Verification items for the finished model (mm, model axes). A direction names the side the tool comes from. Give positions to 0.01 mm unless a question says otherwise; leave off trailing zeros. Write each loop counter-clockwise with the first axis right and the second up, starting at its lowest first coordinate (ties: lowest second). Pieces come first, ordered by that corner, then holes. Notation, with made-up numbers: M -27,-3.5 L 19,-3.5 A23 ccw 19,9.5 Z; hole C 37,10 d7. An arc over 180 degrees is marked long. Answer as a JSON object with one key per item and string values.
Autodesk Fusion 360 part; units mm, degrees
sketch "Sketch1" plane through (0, 0, 0) normal (0, 0, 1) x (1, 0, 0)
  line L0 (36, 27) -> (-36, 27)
  line L1 (-36, 27) -> (-36, -27)
  line L2 (-36, -27) -> (36, -27)
  line L3 (36, -27) -> (36, 27)
  line L4 (36, 30.6) -> (-36, 30.6)
  line L5 (-36, 35.6) -> (-36, -30.6)
  line L6 (-36, -30.6) -> (36, -30.6)
  line L7 (36, -30.6) -> (36, 30.6)
  line L8 (33, 35.6) -> (-36, 35.6)
  line L9 (41, -27.6) -> (41, 27.6)
  line L10 (33, -35.6) -> (-36, -35.6)
  line L11 (-36, -35.6) -> (-36, 30.6)
  arc A0 (41, 27.6) -> (33, 35.6) centre (33, 27.6) ccw
  arc A1 (33, -35.6) -> (41, -27.6) centre (33, -27.6) ccw
  circle A2 centre (-31, 0) radius 1.75
  line L12 (-31, 11) -> (-10, 11)
  arc A3 (-10, 11) -> (-10, 19) centre (-10, 15) ccw
  line L13 (-10, 19) -> (-31, 19)
  arc A4 (-31, 19) -> (-31, 11) centre (-31, 15) ccw
  line L14 (-31, 15) -> (-10, 15) construction
  line L15 (1.75, 0) -> (22.5, 0)
  line L16 (-31, -11) -> (-10, -11)
  line L17 (-10, -19) -> (-31, -19)
  arc A5 (-10, -19) -> (-10, -11) centre (-10, -15) ccw
  arc A6 (-31, -11) -> (-31, -19) centre (-31, -15) ccw
  circle A7 centre (-10, 0) radius 1.75
  dimension "d1" = 72
  dimension "d2" = 54
  dimension "d3" = 61.2
  dimension "d6" = 8
  dimension "d32" = 3.5
  dimension "d34" = 8
  dimension "d40" = 3.5
extrude "Extrude1" add sketch "Sketch1" along normal blind 6.1 contours L3 L4 L5 L6 L7 L8 L9 L10 L11 A0 A1 | L0 L4 L5 L7 L11 | L2 L5 L6 L7 L11
extrude "Extrude2" add sketch "Sketch1" along normal blind 24 contours L3 L4 L5 L6 L7 L8 L9 L10 L11 A0 A1
extrude "Extrude3" add sketch "Sketch1" along normal blind 27 and the other way blind -24
sketch "Sketch2" plane through (0, -35.6, 0) normal (0, -1, 0) x (1, 0, 0)
  line L0 (-36, 0) -> (33, 0)
  line L1 (33, 0) -> (33, 27)
  line L2 (-36, 27) -> (-36, 0)
  line L3 (-36, 0) -> (-49.5029, 27)
  line L4 (-36, 0) -> (-6, 0) construction
  line L5 (-36, 27) -> (-49.5029, 27)
  line L6 (33, 27) -> (-36, 27)
  line L7 (-36, 27) -> (-36, 24)
  line L8 (-36, 24) -> (-36.4845, 24)
  line L9 (-36.4845, 24) -> (-48.0026, 24)
  line L10 (-36, 0) -> (-36, 6.4)
  line L11 (-36, 6.4) -> (-36, 6)
  line L12 (-36, 6.4) -> (-39.2007, 6.4)
  line L13 (-36, 0) -> (-32.4, 0)
  line L14 (-49.5029, 27) -> (-47.5029, 27)
  line L15 (-36, 6.4) -> (-32.4, 6.4)
  line L16 (-32.4, 6.4) -> (-32.4, 0)
  dimension "d11" = 116.57
  dimension "d25" = 6.4
  dimension "d36" = 3.6
  dimension "d37" = 2
extrude "Extrude4" add sketch "Sketch2" against normal blind 5 contours L2 L3 L10 L11 L12 | L2 L3 L8 L9 L12
extrude "Extrude5" add sketch "Sketch2" along normal blind -71.2 and the other way blind 66.2 contours L2 L3 L10 L11 L12 | L2 L3 L8 L9 L12
extrude "Extrude6" add sketch "Sketch2" against normal blind 71.2 contours L2 L3 L5 L7 L8 L9 L14
extrude "Extrude7" cut sketch "Sketch2" along normal blind -8.6 and the other way blind 5 contours L0 L2 L10 L11 L13 L15 L16
extrude "Extrude8" cut sketch "Sketch2" along normal blind -66.2 and the other way blind 62.6 contours L0 L2 L10 L11 L13 L15 L16
chamfer "Chamfer2" distance 1 angle 45 2 edges at (-32.6316, 0.6328, 24) (-11.6316, 0.6328, 24)
sketch "Sketch3" plane through (0, 0, 27) normal (0, 0, 1) x (-1, 0, 0)
  arc A0 (10, 19) -> (10, 11) centre (10, 15) ccw
  line L0 (10, 19) -> (31, 19)
  arc A1 (31, 11) -> (31, 19) centre (31, 15) ccw
  line L1 (31, 11) -> (10, 11)
  circle A2 centre (31, 0) radius 1.75
  circle A3 centre (10, 0) radius 1.75
  arc A4 (31, -19) -> (31, -11) centre (31, -15) ccw
  line L2 (31, -19) -> (10, -19)
  arc A5 (10, -11) -> (10, -19) centre (10, -15) ccw
  line L3 (10, -11) -> (31, -11)
  line L4 (49.5029, 35.6) -> (-33, 35.6)
  arc A6 (-33, 35.6) -> (-41, 27.6) centre (-33, 27.6) ccw
  line L5 (-41, 27.6) -> (-41, -27.6)
  arc A7 (-41, -27.6) -> (-33, -35.6) centre (-33, -27.6) ccw
  line L6 (-33, -35.6) -> (49.5029, -35.6)
  line L7 (49.5029, -35.6) -> (49.5029, 35.6)
  line L8 (2.0837, -40) -> (-45, -40)
  line L9 (-45, -40) -> (-45, 40)
  line L10 (-45, 40) -> (2.0837, 40)
  line L11 (2.0837, 40) -> (2.0837, -40)
extrude "Extrude9" cut sketch "Sketch3" against normal blind 55 contours L4 A6 L5 A7 L6 L11 | L4 A6 L5 A7 L6 L8 L9 L10 L11
chamfer "Chamfer3" distance 1 angle 45 2 edges at (-32.4, -28.8, 6.1) (-32.4, 28.8, 6.1)
1) Thickness scan on L1, parallel to Y at x = -31, z = 26.15; L2, parallel to Y at x = -37.5, z = 16; L3, parallel to Y at x = -17, z = 3.5. Record the ranges inside material, lowest first.
Completed:
{"L1": "y = -35.6 to -19, -11 to -1.75, 1.75 to 11, 19 to 35.6", "L2": "y = -35.6 to -30.6, 30.6 to 35.6", "L3": "y = -35.6 to -27, 27 to 35.6"}
2) Release check for a two-part mould opening along Z. For faces 5 (the face through (-19, -31, 0)), 6 (the face through (-32.4, -29, 3)), 7 (the face through (-17, 29, 6.1)) record: pulls with the +Z half, pulls with the -Z half, needs draft (parallel to the pull), parting line crosses it, or undercut.
Completed:
{"face 5": "pulls with the -Z half", "face 6": "needs draft", "face 7": "undercut"}
3) Go/stop test with flat-tipped pins: pin 1 (4 mm diameter, centred on y = 29, z = 2, fed in from -X); pin 2 (5 mm diameter, centred on x = -41, y = -5, fed in from -Z); pin 3 (3 mm diameter, centred on y = -28.5, z = 1.5, fed in from -X). Record where each tip stops, or that it passes through.
Completed:
{"pin 1": "stops at x = -37.6", "pin 2": "stops at z = 24", "pin 3": "stops at x = -32.4"}
4) Section check A-A on y = -15. Record the boundary of the cut face in (x, z), and give its area (3 significant figures).
Completed:
{"outline": "M -49.5,27 L -48,24 L -35,24 L -35,27 Z; M -6,24 L -2.08,24 L -2.08,27 L -6,27 Z", "area": "53.0 mm2"}
5) Access from +Z, -Z, +X, -X, +Y, -Y to the whole of each face (thin tool, end or side, straight path). Record for faces 1 (the face through (-32.4, 29, 3)), 2 (the face through (-17, -27, 3)), 3 (the face through (-21, -11, 25)), 4 (the face through (-21, -35.6, 14)).
Completed:
{"face 1": "-Z, -X", "face 2": "-Z, +X, -X", "face 3": "+Z, -Z", "face 4": "+Z, -Z, +X, -X, -Y"}
6) Section check D-D on y = 0. Record the boundary of the cut face in (x, z).
Completed:
{"outline": "M -49.5,27 L -48,24 L -33.75,24 L -32.75,25 L -32.75,27 Z; M -29.25,25 L -28.25,24 L -12.75,24 L -11.75,25 L -11.75,27 L -29.25,27 Z; M -8.25,25 L -7.25,24 L -2.08,24 L -2.08,27 L -8.25,27 Z"}
7) Section check C-C on x = -45. Record the boundary of the cut face in (y, z).
Completed:
{"outline": "M -35.6,18 L -30.6,18 L -30.6,24 L 30.6,24 L 30.6,18 L 35.6,18 L 35.6,27 L -35.6,27 Z"}
8) Section check B-B on z = 14. Record the boundary of the cut face in (x, y), and give its area (3 significant figures).
Completed:
{"outline": "M -43,-35.6 L -2.08,-35.6 L -2.08,-30.6 L -43,-30.6 Z; M -43,30.6 L -2.08,30.6 L -2.08,35.6 L -43,35.6 Z", "area": "409 mm2"}
